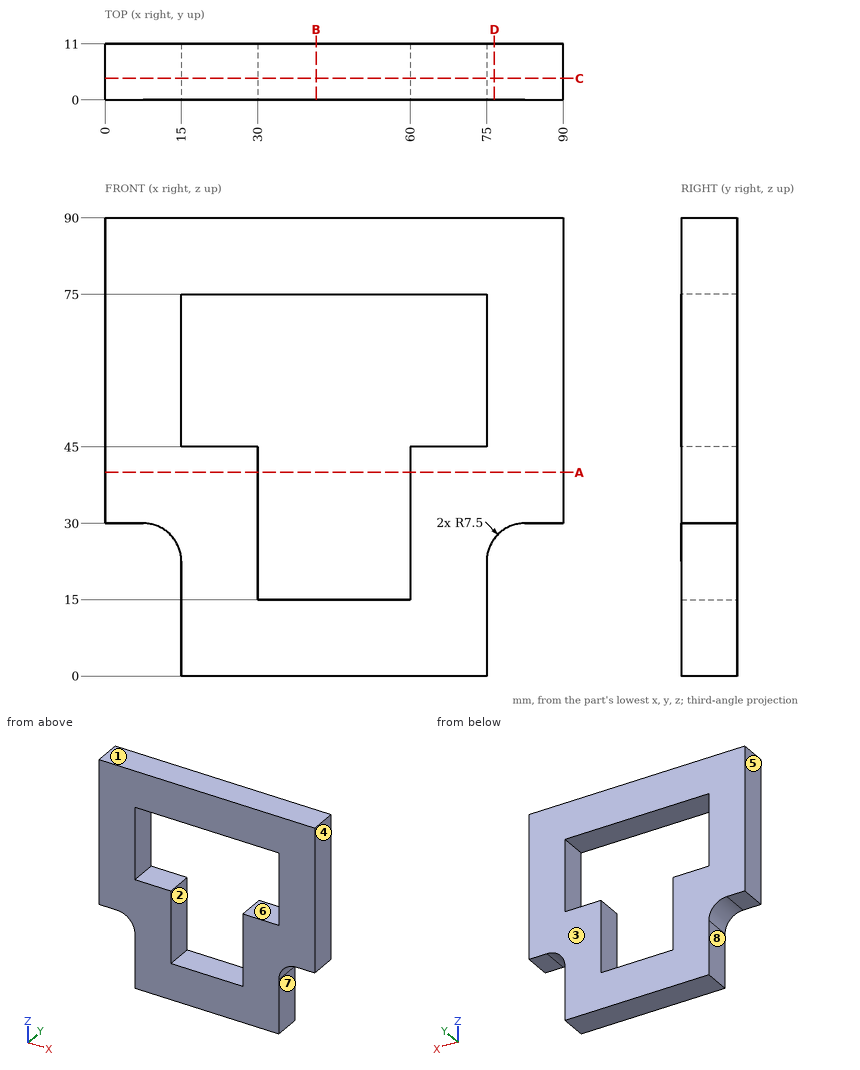
Verification items for this drawing (mm, ordinates from the low corner). A direction names the side the tool comes from. Round coordinates to 2 decimals unless told otherwise and drop trailing zeros. Loops run counter-clockwise (first coordinate to the right, second up) from the corner with the lowest first, then second, coordinate; pieces in that order, holes last. Notation, with made-up numbers: (-32, -4) - (4, -4) arc R32 ccw to (4, 25) - close; hole circle Ø9 at (-29.75, 2.25). An arc over 180 degrees is marked (long way). Answer as CSV lines item,"result". Start each with the question number.
Item 1: Section check B-B (x = 41.5). Record the boundary of the cut face in (y, z), and give its area (3 significant figures).
Item 2: Scan lines: line 1 (Z direction, x = 32.5, y = 4); line 2 (Z direction, x = 64, y = 6.25). Record each from-to range of solid material in increasing order. Write a range as [from, to].
Item 3: Depth check by flat-ended pin: P1, Ø1, axis at y = 1.5, z = 17, coming from the -X side; P2, Ø1.5, axis at x = 11, z = 67, coming from the -Y side; P3, Ø5, axis at x = 80.5, y = 3, coming from the -Z side; P4, Ø4, axis at x = 85.5, y = 7, coming from the -Z side. Enter the tip coordinate at first touch or a pass-through.
Item 4: Section check C-C (y = 4.25). Record the boundary of the cut face in (x, z), and give its area (3 significant figures).
Item 5: Section check D-D (x = 76.5). Record the boundary of the cut face in (y, z).
Item 6: Release check for a two-part mould opening along Z. For the marked faces 1, 2 and 3 record: +Z half, -Z half, draft (parallel to the pull), parting line (faces both ways), or undercut.
Item 7: Section check A-A (z = 40). Record the boundary of the cut face in (x, y), and give its area (3 significant figures).
Item 8: Set-up check for the marked faces 4, 5, 6, 7 and 8: record each of +Z, -Z, +X, -X, +Y, -Y from which the full face is reachable in a straight line by a thin tool's end or side.
Report:
1,outline,"(0, 0) - (11, 0) - (11, 15) - (0, 15) - close; (0, 75) - (11, 75) - (11, 90) - (0, 90) - close"
1,area,"330 mm2"
2,line 1,"z = [0, 15], [75, 90]"
2,line 2,"z = [0, 45], [75, 90]"
3,P1,"stops at x = 15"
3,P2,"stops at y = 0"
3,P3,"stops at z = 28.5"
3,P4,"stops at z = 30"
4,outline,"(0, 30) - (7.5, 30) arc R7.5 cw to (15, 22.5) - (15, 0) - (75, 0) - (75, 22.5) arc R7.5 cw to (82.5, 30) - (90, 30) - (90, 90) - (0, 90) - close; hole (15, 45) - (30, 45) - (30, 15) - (60, 15) - (60, 45) - (75, 45) - (75, 75) - (15, 75) - close"
4,area,"4,520 mm2"
5,outline,"(0, 27) - (11, 27) - (11, 90) - (0, 90) - close"
6,face 1,"+Z half"
6,face 2,"undercut"
6,face 3,"draft"
7,outline,"(0, 0) - (30, 0) - (30, 11) - (0, 11) - close; (60, 0) - (90, 0) - (90, 11) - (60, 11) - close"
7,area,"660 mm2"
8,face 4,"+Z, -Z, +X, +Y, -Y"
8,face 5,"+Z, -Z, -X, +Y, -Y"
8,face 6,"+Y, -Y"
8,face 7,"-Z, +X, +Y, -Y"
8,face 8,"-Z, -X, +Y, -Y"
